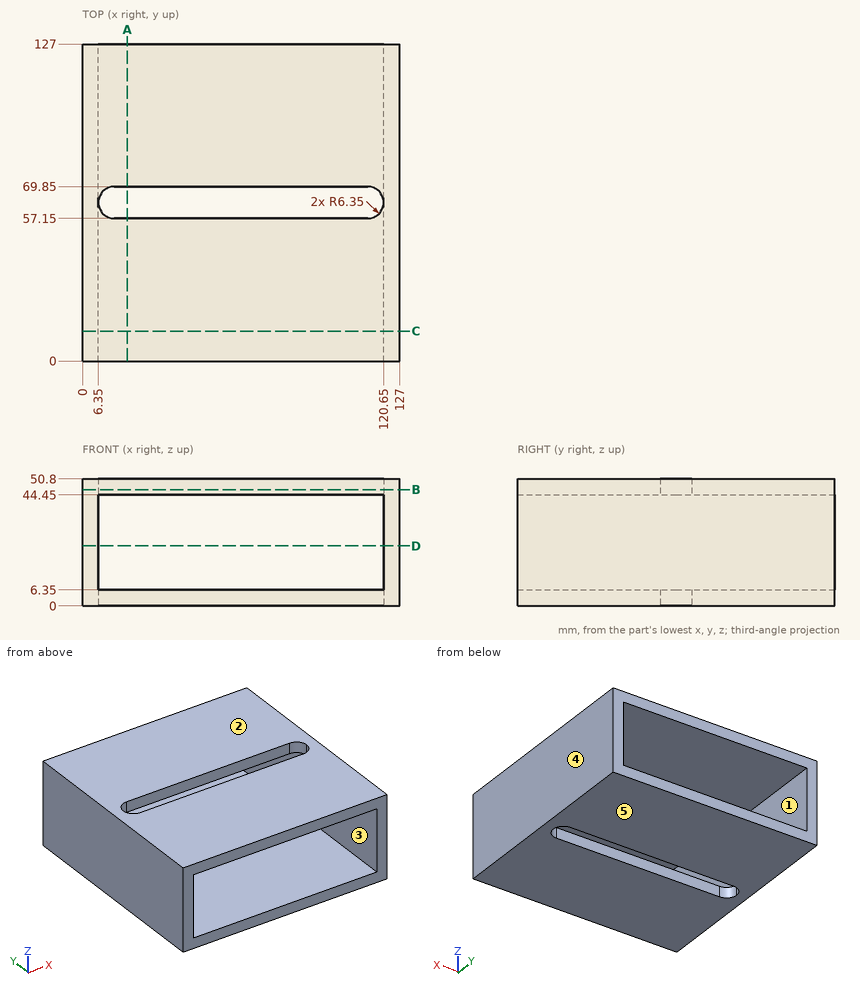
Check sheet for the drawn part. Datum: minimum x, y, z corner. Units: mm. A direction names the side the tool comes from. Round coordinates to 2 decimals unless told otherwise and drop trailing zeros. Loops run counter-clockwise (first coordinate to the right, second up) from the corner with the lowest first, then second, coordinate; pieces in that order, holes last. Notation, with made-up numbers: (-32.5, 27) -> (-25.5, 27) arc R22 ccw to (-25.5, 61) -> close; hole circle Ø9 at (48.5, 87.25). An arc over 180 degrees is marked (long way). Put each result on its own line as item: value. Start each with the question number.
1. Gauge pin test, flat end, axial feed: pin 1 (7 mm diameter, centred on x = 46.5, z = 2, fed in from -Y). Record the tip position at first contact, or that the pin passes through.
2. Draft check along Z on the marked faces 3, 4 and 5. Enter one of: +Z half, -Z half, draft (parallel to the pull), parting line (faces both ways), or undercut.
3. Section check A-A (x = 18). Enter the section's corners in (y, z).
4. Section check C-C (y = 12). Enter the section's corners in (x, z), plus the area to 3 significant figures.
5. Section check D-D (z = 24). Enter the section's corners in (x, y), plus the area to 3 significant figures.
6. Access from +Z, -Z, +X, -X, +Y, -Y to the whole of each face (thin tool, end or side, straight path). Record for the marked faces 1 and 2.
7. Section check B-B (z = 46.5). Enter the section's corners in (x, y), plus the area to 3 significant figures.
8. Scan lines: probe 1 along X at (y, z) = (66, 39.5); probe 2 along Z at (x, y) = (85.5, 100.5); probe 3 along Y at (x, z) = (77, 4). Record each from-to range of solid material in increasing order.
Findings:
1. pin 1: stops at y = 0
2. face 3: undercut
2. face 4: draft
2. face 5: -Z half
3. outline: (0, 0) -> (57.15, 0) -> (57.15, 6.35) -> (0, 6.35) -> close; (0, 44.45) -> (57.15, 44.45) -> (57.15, 50.8) -> (0, 50.8) -> close; (69.85, 0) -> (127, 0) -> (127, 6.35) -> (69.85, 6.35) -> close; (69.85, 44.45) -> (127, 44.45) -> (127, 50.8) -> (69.85, 50.8) -> close
4. outline: (0, 0) -> (127, 0) -> (127, 50.8) -> (0, 50.8) -> close; hole (6.35, 6.35) -> (120.65, 6.35) -> (120.65, 44.45) -> (6.35, 44.45) -> close
4. area: 2,100 mm^2
5. outline: (0, 0) -> (6.35, 0) -> (6.35, 127) -> (0, 127) -> close; (120.65, 0) -> (127, 0) -> (127, 127) -> (120.65, 127) -> close
5. area: 1,610 mm^2
6. face 1: +Y, -Y
6. face 2: +Z, +X, -X, +Y, -Y
7. outline: (0, 0) -> (127, 0) -> (127, 127) -> (0, 127) -> close; hole (12.7, 57.15) -> (114.3, 57.15) arc R6.35 ccw to (114.3, 69.85) -> (12.7, 69.85) arc R6.35 ccw to start
7. area: 14,700 mm^2
8. probe 1: x = 0 to 6.35, 120.65 to 127
8. probe 2: z = 0 to 6.35, 44.45 to 50.8
8. probe 3: y = 0 to 57.15, 69.85 to 127
